The model under review builds one solid part; all positions refer to its coordinate system, in mm. A direction names the side the tool comes from. Round coordinates to 2 decimals unless told otherwise and drop trailing zeros. Loops run counter-clockwise (first coordinate to the right, second up) from the corner with the lowest first, then second, coordinate; pieces in that order, holes last. Notation, with made-up numbers: M -0.5,30 L 45.5,30 A15 cw 45.5,58 Z; hole C 24,-37.5 d11. An arc over 180 degrees is marked long. Answer as a JSON object with one key per item and string values. Group by question number.
Item 1: To check wall thickness, follow line 1 (Y direction, x = 127.5, z = -500); line 2 (Y direction, x = -54.5, z = -507); line 3 (X direction, y = -17, z = 680.5). State the ranges of each line that lie inside material, in increasing order.
Item 2: Consider section A-A (z = -500). Give the boundary of the cut face in (x, y), and give its area (3 significant figures).
Item 3: Consider section C-C (y = 522). Give the boundary of the cut face in (x, z).
Item 4: Consider section B-B (x = -281). Give the boundary of the cut face in (y, z).
Item 5: Consider section D-D (y = 230). Give the boundary of the cut face in (x, z).
Item 6: Insertion check: P1, Ø5, axis at x = -42, y = 643, coming from the +Z side; P2, Ø2, axis at y = 196, z = -345, coming from the -X side; P3, Ø4, axis at x = -93, z = 493.5, coming from the +Y side. Each pin has a flat end and moves straight along its axis. Give the tip position at first contact, or say it passes through.
Item 7: Tool access review of faces 4 (the face through (-439, 60, 11)), 5 (the face through (-4, 60, 11)), 6 (the face through (-218, 180, 307)), 7 (the face through (222, 180, 307)), 8 (the face through (380, 326, -293)): name each direction out of +Z, -Z, +X, -X, +Y, -Y from which nothing blocks a thin tool from reaching the whole face with its end or side.
Item 8: The part is to be moulded in two halves that separate along Y. For faces 1 (the face through (260, 1, 11)), 2 (the face through (-382, -60, 11)), 3 (the face through (5.32, 645.06, -643.07)), say which applies: +Y half, -Y half, draft (parallel to the pull), parting line (faces both ways), or undercut.
```python
from build123d import *

# Parameters (mm, degrees)
BOSS_EXTRUDE1_DEPTH = 800
SKETCH2_R           = 150
BOSS_EXTRUDE5_DEPTH = 760
RIB1_REACH          = 1305.84
SKETCH4_WALL_W      = 3904.804378638
SKETCH4_WALL_H      = 120


with BuildPart() as part:
    # Sketch1 → Boss-Extrude1 (new, symmetric)
    with BuildSketch(Plane.XY):
        Polygon((380, 60), (260, 60), (260, -60), (500, -60), (500, 60), align=None)
        Polygon((-380, 180), (-380, 60), (-260, 60), (260, 60), (380, 60), (380, 180), align=None)
        Polygon((-260, 60), (-380, 60), (-500, 60), (-500, -60), (-260, -60), align=None)
    extrude(amount=BOSS_EXTRUDE1_DEPTH, both=True)

    # Sketch2 → Boss-Extrude5 (add)
    with BuildSketch(Plane(origin=(380, 0, 0), x_dir=(0, 0, -1), z_dir=(1, 0, 0))):
        with BuildLine():
            Line((800, 180), (800, 600))
            ThreePointArc((800, 600), (500, 900), (200, 600))
            Line((200, 600), (200, 180))
            Line((200, 180), (800, 180))
        make_face()
        with Locations((500, 600)):
            Circle(SKETCH2_R, mode=Mode.SUBTRACT)
    extrude(amount=-BOSS_EXTRUDE5_DEPTH)

    # Sketch4 wall → Rib1 (add, up to next)
    with BuildSketch(Plane(origin=(0, 508.510499954, 241.952495347), x_dir=(0, 0.507303776233, -0.861767299576), z_dir=(0, 0.861767299576, 0.507303776233)), mode=Mode.PRIVATE) as rib1_sk1:
        Rectangle(SKETCH4_WALL_W, SKETCH4_WALL_H)
    rib1_tool1 = extrude(rib1_sk1.sketch, amount=-RIB1_REACH, mode=Mode.PRIVATE) - part.part
    add(rib1_tool1.solids().sort_by_distance((0, 508.510499954, 241.952495347))[0])


solid = part.part
```
Geometry results:
{
 "1": {"line 1": "y = 60 to 450, 750 to 900", "line 2": "y = 60 to 450.16, 749.84 to 899.92", "line 3": "x = -500 to -260, 260 to 500"},
 "2": {"outline": "M -500,-60 L -260,-60 L -260,60 L 260,60 L 260,-60 L 500,-60 L 500,60 L 380,60 L 380,450 L -380,450 L -380,60 L -500,60 Z; M -380,750 L 380,750 L 380,900 L -380,900 Z", "area": "468,000 mm^2"},
 "3": {"outline": "M -380,-800 L 380,-800 L 380,-628.12 L -380,-628.12 Z; M -380,-371.88 L 380,-371.88 L 380,-200 L 60,-200 L 60,219.04 L -60,219.04 L -60,-200 L -380,-200 Z"},
 "4": {"outline": "M -60,-800 L 600,-800 A300 ccw 600,-200 L 180,-200 L 180,800 L -60,800 Z; hole C 600,-500 d300"},
 "5": {"outline": "M -380,-800 L 380,-800 L 380,-200 L 60,-200 L 60,715.06 L -60,715.06 L -60,-200 L -380,-200 Z"},
 "6": {"P1": "stops at z = 17.74", "P2": "stops at x = -380", "P3": "stops at y = 180"},
 "7": {"face 4": "+Z, -Z, -X, +Y", "face 5": "+Z, -Z, -Y", "face 6": "+Z, -X, +Y", "face 7": "+Z, +X, +Y", "face 8": "+Z, -Z, +X, +Y"},
 "8": {"face 1": "draft", "face 2": "-Y half", "face 3": "undercut"}
}
